```python
from build123d import *

# Parameters (mm, degrees)
BOSS_EXTRUDE1_DEPTH = 33.2486
BOSS_EXTRUDE1_TAPER = -26.56505118
SKETCH2_OUTSIDE_W   = 117.17
SKETCH2_OUTSIDE_H   = 114.076
CUT_EXTRUDE1_DEPTH  = 33.2486
CUT_EXTRUDE1_TAPER  = 26.56505118
SCALE1_SCALE        = 1.125
SKETCH3_W           = 93.211542344
SKETCH3_H           = 68.986167311
CUT_EXTRUDE2_DEPTH  = 19.7023376
SHELL1_T            = -2.54


with BuildPart() as part:
    # Sketch1 → Boss-Extrude1 (new body)
    with BuildSketch(Plane(origin=(0, 0, 0), x_dir=(1, 0, 0), z_dir=(0, 1, 0))):
        Polygon((12.078417757, 3.924515829), (0, 12.7), (-12.078417757, 3.924515829), (-7.464872704, -10.274515829), (7.464872704, -10.274515829), align=None)
    extrude(amount=BOSS_EXTRUDE1_DEPTH, taper=BOSS_EXTRUDE1_TAPER)

    # Sketch2 outside → Cut-Extrude1 (cut)
    with BuildSketch(Plane(origin=(0, 33.2486, 0), x_dir=(1, 0, 0), z_dir=(0, 1, 0))):
        with Locations((0, 3.175)):
            Rectangle(SKETCH2_OUTSIDE_W, SKETCH2_OUTSIDE_H)
        Polygon((7.464872704, 10.274515829), (-7.464872704, 10.274515829), (-12.078417757, -3.924515829), (0, -12.7), (12.078417757, -3.924515829), align=None, mode=Mode.SUBTRACT)
    extrude(amount=-CUT_EXTRUDE1_DEPTH, taper=CUT_EXTRUDE1_TAPER, mode=Mode.SUBTRACT)


with BuildPart() as part_1:
    # Scale1: scaled about (0, 0, 0)
    add(part.part.scale(SCALE1_SCALE))

    # Sketch3 → Cut-Extrude2 (cut, through all)
    with BuildSketch(Plane(origin=(0, 18.7023375, 0), x_dir=(1, 0, 0), z_dir=(0, 1, 0))):
        with Locations((6.510218593, 0.168740009)):
            Rectangle(SKETCH3_W, SKETCH3_H)
    extrude(amount=CUT_EXTRUDE2_DEPTH, mode=Mode.SUBTRACT)

    # Shell1
    shell1_openings = [part_1.faces().sort_by_distance(p)[0] for p in [
        (0, 18.7023375, 0),
    ]]
    offset(amount=SHELL1_T, openings=shell1_openings, kind=Kind.INTERSECTION)


solid = part_1.part
```
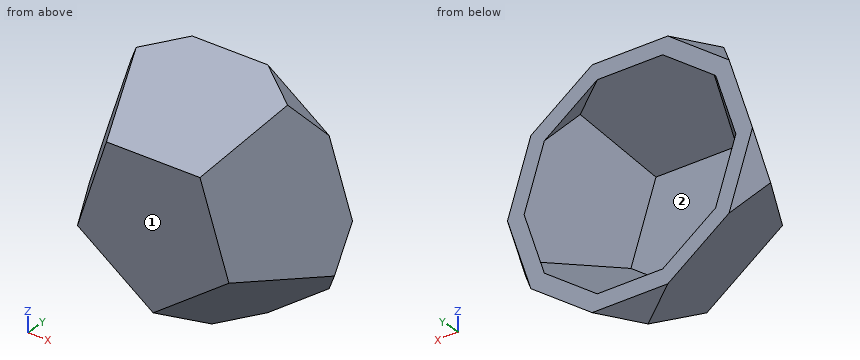
The model under review builds one solid part; all positions refer to its coordinate system, in mm. Face numbers are marked on the shaded views. Round coordinates to 2 decimals unless told otherwise and drop trailing zeros. Put each result on its own line as item: value.
Q1. Mouldability with a two-part tool opening along Z and no side actions: class the marked faces 1 and 2 as released by +Z, released by -Z, zero draft, split by the parting line, or undercut.
Result set:
face 1: zero draft
face 2: undercut
Q2. To check wall thickness, follow L1, parallel to Y at x = -5.5, z = 8; L2, parallel to Z at x = 0, y = 17.75; L3, parallel to X at y = 10.25, z = 8. State the ranges of each line that lie inside material, in increasing order.
Result set:
L1: y = 0 to 2.54
L2: z = -21.39 to -18.55, 17.59 to 20.43
L3: x = -14.94 to -11.96, 11.96 to 14.94
Q3. For pin 1 (3 mm diameter, centred on y = 10.5, z = -8.5, fed in from -X); pin 2 (1.5 mm diameter, centred on x = -4.5, z = -1.5, fed in from -Y); pin 3 (8 mm diameter, centred on y = 6.5, z = -8, fed in from +X); pin 4 (6 mm diameter, centred on y = 11.5, z = 7, fed in from -X), all flat-tipped, find the tip position at first contact; note any pin that passes through.
Result set:
pin 1: stops at x = -19.32
pin 2: stops at y = 0
pin 3: stops at x = 19.55
pin 4: stops at x = -17.78
